Could you check a few things on this model? Use its own coordinates, in mm. Face numbers are marked on the shaded views. A direction names the side the tool comes from. Give positions to 0.01 mm unless a question says otherwise; leave off trailing zeros. Loops run counter-clockwise (first coordinate to the right, second up) from the corner with the lowest first, then second, coordinate; pieces in that order, holes last. Notation, with made-up numbers: (65, 63) -> (122, 63) arc R13 cw to (122, 70) -> close; hole circle Ø8 at (74.25, 28.5). An arc over 180 degrees is marked (long way). Write each question's results on one line, items separated by ' | '. Start each with the question number.
Q1. Will these pins go through, and if not, where does the flat tip stop? P1, Ø3, axis at x = -5, z = -17.5, coming from the +Y side; P2, Ø5, axis at x = 13.2, z = 22, coming from the +Y side; P3, Ø4, axis at y = 7.5, z = 11.5, coming from the -X side; P4, Ø2, axis at x = 13.2, z = 22, coming from the -Y side.
Q2. If we section it at D-D, the plane x = -7.75: List the corners of the cut face in (y, z) for me.
Q3. Which directions (+Z, -Z, +X, -X, +Y, -Y) give clear straight access to the entire face, cutting with the end or side of a thin tool? Please do the marked faces 1, 2, 3, 4 and 5.
Q4. If we section it at B-B, the plane z = -2: List the corners of the cut face in (x, y) for me.
Q5. If we section it at C-C, the plane z = -16.5: List the corners of the cut face in (x, y) for me.
Q6. We'd pull the mould along Z, two halves only. Please class the marked faces 6, 7 and 8: released by +Z, released by -Z, zero draft, split by the parting line, or undercut.
Q7. If we section it at A-A, the plane y = 6: List the corners of the cut face in (x, z) for me, plus the area to 3 significant figures.
Q8. If I drill on line 1 along Z through (x, y) = (13.2, -4.5); line 2 along Z through (x, y) = (13.2, 5.7); line 3 along X through (y, z) = (3.75, 12.5), over which ranges is the centre line in solid material (lowest first)?
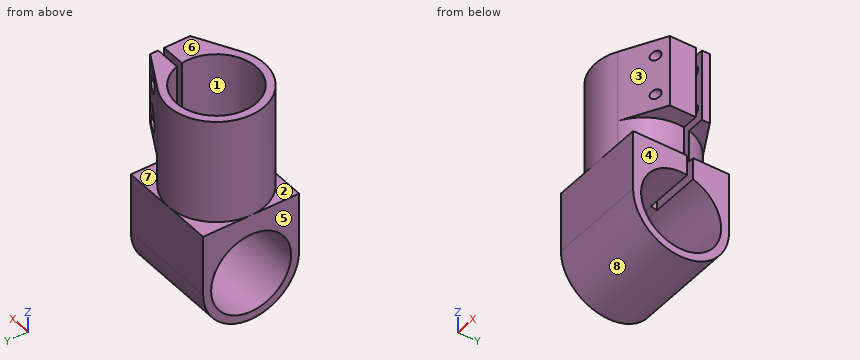
from build123d import *

# Parameters (mm, degrees)
BOSS_EXTRU_1_DEPTH           = 26
BOSS_EXTRU_4_DEPTH           = 25
ESQUISSE5_R                  = 17.691806013
ESQUISSE5_R_2                = 12
ENL_V_MAT_EXTRU_2_DEPTH      = 8
ENL_V_START                  = -2
ESQUISSE6_R                  = 3
ENL_V_MAT_EXTRU_3_DEPTH      = 33.785054262
ESQUISSE7_R                  = 1.5
ENL_V_MAT_EXTRU_4_DEPTH      = 2
ENL_V_MAT_EXTRU_5_DEPTH      = 35.165040612
ENL_V_MAT_EXTRU_5_DEPTH_BACK = 35.165040612
ESQUISSE8_R                  = 1.2
ESQUISSE9_R                  = 10
BOSS_EXTRU_5_DEPTH           = 12.5


with BuildPart() as part:
    # Esquisse1 → Boss.-Extru.1 (new body)
    with BuildSketch(Plane.XY):
        with BuildLine():
            Line((5.700064076, 10.559794957), (16, 5))
            Line((16, 5), (16, 3))
            Line((16, 3), (9.539392014, 3))
            ThreePointArc((9.539392014, 3), (-9.742038622, -2.256697475), (9.886859967, 1.5))
            Line((9.886859967, 1.5), (16, 1.5))
            Line((16, 1.5), (16, -5))
            Line((16, -5), (5.700064076, -10.559794957))
            ThreePointArc((5.700064076, -10.559794957), (-12, 0), (5.700064076, 10.559794957))
        make_face()
    extrude(amount=BOSS_EXTRU_1_DEPTH)

    # Esquisse2 → Boss.-Extru.4 (add)
    with BuildSketch(Plane(origin=(-12, 0, 0), x_dir=(0, 0, -1), z_dir=(1, 0, 0))):
        with BuildLine():
            Line((0, -12), (15, -12))
            ThreePointArc((15, -12), (27, 0), (15, 12))
            Line((15, 12), (0, 12))
            Line((0, 12), (0, 3))
            Line((0, 3), (5.460607986, 3))
            ThreePointArc((5.460607986, 3), (24.742038622, -2.256697475), (5.113140033, 1.5))
            Line((5.113140033, 1.5), (0, 1.5))
            Line((0, 1.5), (0, -12))
        make_face()
    extrude(amount=BOSS_EXTRU_4_DEPTH)

    # Esquisse5 → Enlèv. mat.-Extru.2 (cut)
    with BuildSketch(Plane.XY):
        Circle(ESQUISSE5_R)
        Circle(ESQUISSE5_R_2, mode=Mode.SUBTRACT)
    extrude(amount=ENL_V_MAT_EXTRU_2_DEPTH, mode=Mode.SUBTRACT)

    # Esquisse6 → Enlèv. mat.-Extru.3 (cut, through all)
    with BuildSketch(Plane(origin=(0, 3, 0), x_dir=(-1, 0, 0), z_dir=(0, -1, 0)).offset(ENL_V_START)):
        with Locations((-13.2, -12)):
            Circle(ESQUISSE6_R)
        with Locations((-13.2, -22)):
            Circle(ESQUISSE6_R)
    extrude(amount=-ENL_V_MAT_EXTRU_3_DEPTH, mode=Mode.SUBTRACT)

    # Esquisse7 → Enlèv. mat.-Extru.4 (cut)
    with BuildSketch(Plane(origin=(0, 5, 0), x_dir=(1, 0, 0), z_dir=(0, 1, 0))):
        with Locations(Location((13.2, -12, 0), (0, 0, 270))):
            Circle(ESQUISSE7_R)
        with Locations(Location((13.2, -22, 0), (0, 0, 270))):
            Circle(ESQUISSE7_R)
    extrude(amount=-ENL_V_MAT_EXTRU_4_DEPTH, mode=Mode.SUBTRACT)

    # Esquisse8 → Enlèv. mat.-Extru.5 (cut, two sides: drawn at the far end of the back side and taken through both)
    with BuildSketch(Plane(origin=(0, 1.5, 0), x_dir=(1, 0, 0), z_dir=(0, 1, 0)).offset(-ENL_V_MAT_EXTRU_5_DEPTH_BACK)):
        with Locations((13.2, -12)):
            Circle(ESQUISSE8_R)
        with Locations((13.2, -22)):
            Circle(ESQUISSE8_R)
    extrude(amount=ENL_V_MAT_EXTRU_5_DEPTH + ENL_V_MAT_EXTRU_5_DEPTH_BACK, mode=Mode.SUBTRACT)

    # Esquisse9 → Boss.-Extru.5 (add)
    with BuildSketch(Plane.ZY.offset(12)):
        with BuildLine():
            Line((-15, 12), (0, 12))
            Line((0, 12), (0, -12))
            Line((0, -12), (-15, -12))
            ThreePointArc((-15, -12), (-27, 0), (-15, 12))
        make_face()
        with Locations((-15, 0)):
            Circle(ESQUISSE9_R, mode=Mode.SUBTRACT)
    extrude(amount=-BOSS_EXTRU_5_DEPTH)


solid = part.part
Final values:
1) P1: stops at y = 11.96 | P2: stops at y = 5 | P3: stops at x = -10.67 | P4: passes through
2) outline: (-12, -15) arc R12 ccw to (12, -15) -> (12, 0) -> (9.16, 0) -> (9.16, 26) -> (6.32, 26) -> (6.32, 0) -> (-6.32, 0) -> (-6.32, 26) -> (-9.16, 26) -> (-9.16, 0) -> (-12, 0) -> close; hole circle Ø20 at (0, -15)
3) face 1: +Z | face 2: +Z, -X, -Y | face 3: +Z, +X, -Y | face 4: -Z, +X, +Y, -Y | face 5: +Z, -Z, -X, +Y, -Y
4) outline: (-12, -12) -> (13, -12) -> (13, 1.5) -> (0.5, 1.5) -> (0.5, 3) -> (13, 3) -> (13, 12) -> (-12, 12) -> close
5) outline: (-12, -11.91) -> (13, -11.91) -> (13, -9.89) -> (-12, -9.89) -> close; (-12, 9.89) -> (13, 9.89) -> (13, 11.91) -> (-12, 11.91) -> close
6) face 6: released by +Z | face 7: undercut | face 8: released by -Z
7) outline: (-12, -25.39) -> (13, -25.39) -> (13, -23) -> (-12, -23) -> close; (-12, -7) -> (13, -7) -> (13, 0) -> (10.39, 0) -> (10.39, 8) -> (14.15, 8) -> (14.15, 9.15) arc R3 cw (long way) to (14.15, 14.85) -> (14.15, 19.15) arc R3 cw (long way) to (14.15, 24.85) -> (14.15, 26) -> (8, 26) -> (8, 0) -> (-8, 0) -> (-8, 26) -> (-10.39, 26) -> (-10.39, 0) -> (-12, 0) -> close | area: 387 mm²
8) line 1: z = 8 to 10.8, 13.2 to 20.8, 23.2 to 26 | line 2: z = 8 to 9, 15 to 19, 25 to 26 | line 3: x = -11.4 to -9.27, 9.27 to 11.79, 14.61 to 16
